from build123d import *

# Parameters (mm, degrees)
BOSS_EXTRUDE1_DEPTH = 431.8
SKETCH4_W           = 15.875
SKETCH4_H           = 25.4
CUT_EXTRUDE1_DEPTH  = 6.35
SKETCH5_W           = 1.5875
SKETCH5_H           = 25.4
CUT_EXTRUDE2_DEPTH  = 6.35
SKETCH6_R           = 1.4224
CUT_EXTRUDE3_DEPTH  = 5.08
CUT_EXTRUDE4_START  = -2.54
CUT_EXTRUDE4_DEPTH  = 2.54
SKETCH8_R           = 1.4224
CUT_EXTRUDE5_DEPTH  = 5.08
SKETCH9_W           = 28.861002292
SKETCH9_H           = 547.524656259
CUT_EXTRUDE6_DEPTH  = 30.48
CUT_EXTRUDE7_START  = -3.175
CUT_EXTRUDE7_DEPTH  = 3.175


# Read off the part's stored shape, not the designer's step: Cut-Extrude7
with BuildPart() as part:
    # Sketch2 → Boss-Extrude1 (new body)
    with BuildSketch(Plane(origin=(0, 0, 0), x_dir=(1, 0, 0), z_dir=(0, 1, 0))):
        with BuildLine():
            Line((0, 0), (19.05, 0))
            Line((19.05, 0), (19.05, 1.5875))
            ThreePointArc((19.05, 1.5875), (18.585032015, 2.710032015), (17.4625, 3.175))
            Line((17.4625, 3.175), (4.7625, 3.175))
            ThreePointArc((4.7625, 3.175), (3.639967985, 3.639967985), (3.175, 4.7625))
            Line((3.175, 4.7625), (3.175, 17.4625))
            ThreePointArc((3.175, 17.4625), (2.710032015, 18.585032015), (1.5875, 19.05))
            Line((1.5875, 19.05), (0, 19.05))
            Line((0, 19.05), (0, 0))
        make_face()
    extrude(amount=BOSS_EXTRUDE1_DEPTH)

    # Sketch4 → Cut-Extrude1 (cut)
    with BuildSketch(Plane(origin=(3.175, 0, 0), x_dir=(0, 0, -1), z_dir=(1, 0, 0))):
        with Locations((11.1125, 419.1)):
            Rectangle(SKETCH4_W, SKETCH4_H)
    extrude(amount=-CUT_EXTRUDE1_DEPTH, mode=Mode.SUBTRACT)

    # Sketch5 → Cut-Extrude2 (cut)
    with BuildSketch(Plane.ZY.offset(-3.175)):
        with Locations((-3.96875, 419.1)):
            Rectangle(SKETCH5_W, SKETCH5_H)
    extrude(amount=-CUT_EXTRUDE2_DEPTH, mode=Mode.SUBTRACT)

    # Sketch6 → Cut-Extrude3 (cut)
    with BuildSketch(Plane(origin=(3.175, 0, 0), x_dir=(0, 0, -1), z_dir=(1, 0, 0))):
        with Locations((11.1125, 109.5375)):
            Circle(SKETCH6_R)
        with Locations((11.1125, 203.2)):
            Circle(SKETCH6_R)
        with Locations((11.1125, 296.8625)):
            Circle(SKETCH6_R)
        with Locations((11.1125, 11.1125)):
            Circle(SKETCH6_R)
        with Locations((11.1125, 395.2875)):
            Circle(SKETCH6_R)
    extrude(amount=-CUT_EXTRUDE3_DEPTH, mode=Mode.SUBTRACT)

    # Sketch7 → Cut-Extrude4 (cut)
    with BuildSketch(Plane(origin=(0, 431.8, 0), x_dir=(1, 0, 0), z_dir=(0, 1, 0)).offset(CUT_EXTRUDE4_START)):
        with BuildLine():
            Line((17.4625, 3.175), (0, 3.175))
            Line((0, 3.175), (0, 0))
            Line((0, 0), (19.05, 0))
            Line((19.05, 0), (19.05, 1.5875))
            ThreePointArc((19.05, 1.5875), (18.585032015, 2.710032015), (17.4625, 3.175))
        make_face()
    extrude(amount=CUT_EXTRUDE4_DEPTH, mode=Mode.SUBTRACT)

    # Sketch8 → Cut-Extrude5 (cut)
    with BuildSketch(Plane(origin=(0, 0, -3.175), x_dir=(-1, 0, 0), z_dir=(0, 0, -1))):
        with Locations((-9.525, 419.735)):
            Circle(SKETCH8_R)
        with Locations((-9.525, 414.02)):
            Circle(SKETCH8_R)
    extrude(amount=-CUT_EXTRUDE5_DEPTH, mode=Mode.SUBTRACT)


with BuildPart() as body_2:
    # Mirror3: mirrored copy
    add(part.part.mirror(Plane.XY.offset(2.54)))

    # Cut-Extrude7 outline → Cut-Extrude7 (cut)
    with BuildSketch(Plane.XY.offset(8.255).offset(CUT_EXTRUDE7_START)):
        with BuildLine():
            ThreePointArc((0, 419.735), (2.789807909, 426.470192091), (9.525, 429.26))
            Line((9.525, 429.26), (0, 429.26))
            Line((0, 429.26), (0, 419.735))
        make_face()
        with BuildLine():
            ThreePointArc((9.525, 429.26), (16.260192091, 426.470192091), (19.05, 419.735))
            Line((19.05, 419.735), (19.05, 429.26))
            Line((19.05, 429.26), (9.525, 429.26))
        make_face()
    extrude(amount=CUT_EXTRUDE7_DEPTH, mode=Mode.SUBTRACT)


with BuildPart() as part_1:
    add(part.part)

    # Sketch9 → Cut-Extrude6 (cut)
    with BuildSketch(Plane.XY.offset(2.54)):
        with Locations((7.805746781, 195.778589833)):
            Rectangle(SKETCH9_W, SKETCH9_H)
    extrude(amount=-CUT_EXTRUDE6_DEPTH, mode=Mode.SUBTRACT)


solid = body_2.part
Read the model definition and answer for the solid it produces. Units are mm, in the model's axes. A direction names the side the tool comes from. Give positions to 0.01 mm unless a question says otherwise; leave off trailing zeros. Use a Markdown table: item, result.
Q1. Find the intervals of material crossed by line 1 along Y through (x, z) = (1.5, 17.25); line 2 along Z through (x, y) = (4.25, 396); line 3 along X through (y, z) = (17, 18.25) (3 decimals), in increasing order.
Solved:
| item | result |
|---|---|
| line 1 | y = 0 to 10.16, 12.06 to 108.59, 110.49 to 202.25, 204.15 to 295.91, 297.81 to 394.34, 396.24 to 406.4 |
| line 2 | z = 5.08 to 8.34 |
| line 3 | x = 0 to 3.175 |
Q2. Each of these flat-tipped pins is pushed along its axis until it touches: pin 1 (3.5 mm diameter, centred on y = 203.2, z = 16.19, fed in from +X) (3 decimals); pin 2 (1.5 mm diameter, centred on x = 6.5, y = 172.5, fed in from +Z) (3 decimals); pin 3 (10 mm diameter, centred on y = 247, z = 14, fed in from +X). Where does it stop, or does it pass through?
Solved:
| item | result |
|---|---|
| pin 1 | stops at x = 3.175 |
| pin 2 | stops at z = 8.255 |
| pin 3 | stops at x = 3.42 |
Q3. A tool of negligible diameter and unlimited length cuts with its end or side. For faces 1 (the face through (0, 207, 15)), 2 (the face through (3.175, 200, 16)), from which of +Z, -Z, +X, -X, +Y, -Y can it reach the whole face along a straight path? Write none if from no direction.
Solved:
| item | result |
|---|---|
| face 1 | +Z, -Z, -X, +Y, -Y |
| face 2 | +Z, +X, +Y, -Y |
